Work out the finished part from the listing and answer in its coordinate system (mm). Face numbers are marked on the shaded views. A direction names the side the tool comes from. Coordinates: 2 decimals unless noted, no trailing zeros. Order: outer loops, then holes, each group sorted by start corner. A loop starts at its lowest first (then second) coordinate and runs counter-clockwise, first axis right, second up. Notation, with made-up numbers: M 22,22.25 L 36,22.25 A14 ccw 36,33.25 Z; hole C 68,-29.5 d5. An arc over 180 degrees is marked long. Use a Markdown table: item, result.
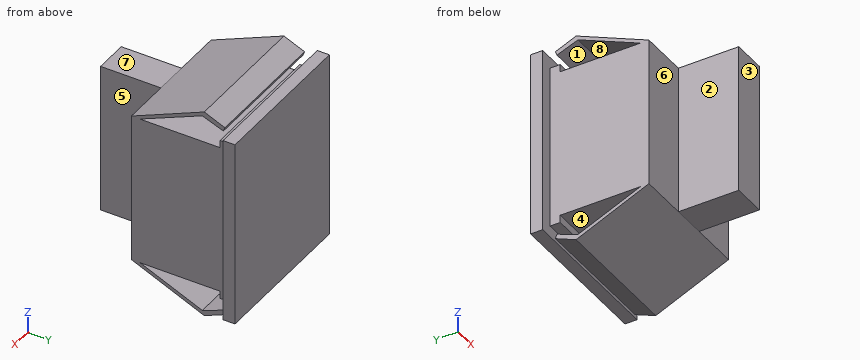
from build123d import *

# Parameters (mm, degrees)
EXTRUDE_1_DEPTH          = 25.6
SKETCH_2_OUTSIDE_W       = 38.032
SKETCH_2_OUTSIDE_H       = 40.832
CUT_EXTRUDE_1_DEPTH      = 6.235907328
CUT_EXTRUDE_1_DEPTH_BACK = 31.235907328


with BuildPart() as part:
    # Эскиз1 → Бобышка-Вытянуть1 (new body)
    with BuildSketch(Plane(origin=(0, 0, 0), x_dir=(0, 0, -1), z_dir=(1, 0, 0))):
        Polygon((12.5, 0), (-12.5, 0), (-12.5, 10), (-17.735907328, 22.085646779), (-16.27222348, 25.510475942), (-15.6, 25.25148825), (-16.94444696, 21.761867538), (-12.5, 11.400931817), (-12.5, 24.709221845), (-13.75, 24.709221845), (-13.75, 26.4), (-15.6, 26.4), (-15.6, 28.4), (15.6, 28.4), (15.6, 26.4), (13.75, 26.4), (13.75, 24.709221845), (12.5, 24.709221845), (12.5, 11.400931817), (16.94444696, 21.761867538), (15.6, 25.25148825), (16.27222348, 25.510475942), (17.735907328, 22.085646779), (12.5, 10), align=None)
    extrude(amount=EXTRUDE_1_DEPTH)

    # Эскиз2 outside → Вырез-Вытянуть1 (cut, two sides)
    with BuildSketch(Plane.XY.offset(12.5)) as cut_extrude_1_sk:
        with Locations((12.8, 14.2)):
            Rectangle(SKETCH_2_OUTSIDE_W, SKETCH_2_OUTSIDE_H)
        Polygon((2, 10), (2, 26.4), (0, 26.4), (0, 28.4), (25.6, 28.4), (25.6, 26.4), (23.6, 26.4), (23.6, 10), (15.6, 10), (15.6, 0), (10, 0), (10, 10), align=None, mode=Mode.SUBTRACT)
    extrude(amount=CUT_EXTRUDE_1_DEPTH, mode=Mode.SUBTRACT)
    extrude(cut_extrude_1_sk.sketch, amount=-CUT_EXTRUDE_1_DEPTH_BACK, mode=Mode.SUBTRACT)


solid = part.part
1. For the marked faces 5, 6, 7 and 8, determine the directions among +Z, -Z, +X, -X, +Y, -Y from which every point of the face is accessible in a straight line to the end or side of a thin tool.
Answers below:
| item | result |
|---|---|
| face 5 | +Z, -Z, +X, -Y |
| face 6 | +Z, -Z, -X, -Y |
| face 7 | +Z, +X, -X, -Y |
| face 8 | +X, -X |
2. Section D-D on z = 0 is taken. Determine the outline of the cut face in (x, y).
Answers below:
| item | result |
|---|---|
| outline | M 0,26.4 L 2,26.4 L 2,10 L 10,10 L 10,0 L 15.6,0 L 15.6,10 L 23.6,10 L 23.6,26.4 L 25.6,26.4 L 25.6,28.4 L 0,28.4 Z |
3. Flat-ended cylindrical pins translate along their axes: P1, Ø3, axis at y = 22, z = 9.5, coming from the -X side; P2, Ø0.6, axis at x = 16.5, y = 27.5, coming from the +Z side; P3, Ø6, axis at y = 3, z = 5.5, coming from the -X side; P4, Ø6.5, axis at x = 18.5, z = 3, coming from the -Y side. Find the tip coordinate at first contact, or state that the pin passes through.
Answers below:
| item | result |
|---|---|
| P1 | x = 2 |
| P2 | z = 15.6 |
| P3 | x = 10 |
| P4 | y = 0 |
4. For a pull along Y with two mould halves and no side action, classify the marked faces 1, 2, 3 and 4 as +Y half, -Y half, draft (parallel to the pull), parting line (faces both ways), or undercut.
Answers below:
| item | result |
|---|---|
| face 1 | undercut |
| face 2 | draft |
| face 3 | -Y half |
| face 4 | undercut |
5. Section C-C on y = 18.25 is taken. Determine the outline of the cut face in (x, z).
Answers below:
| item | result |
|---|---|
| outline | M 2,-16.07 L 23.6,-16.07 L 23.6,-15.44 L 2,-15.44 Z; M 2,-12.5 L 23.6,-12.5 L 23.6,12.5 L 2,12.5 Z; M 2,15.44 L 23.6,15.44 L 23.6,16.07 L 2,16.07 Z |
6. Section B-B on x = 14.25 is taken. Determine the outline of the cut face in (y, z).
Answers below:
| item | result |
|---|---|
| outline | M 0,-12.5 L 10,-12.5 L 22.09,-17.74 L 25.51,-16.27 L 25.25,-15.6 L 21.76,-16.94 L 11.4,-12.5 L 24.71,-12.5 L 24.71,-13.75 L 26.4,-13.75 L 26.4,-15.6 L 28.4,-15.6 L 28.4,15.6 L 26.4,15.6 L 26.4,13.75 L 24.71,13.75 L 24.71,12.5 L 11.4,12.5 L 21.76,16.94 L 25.25,15.6 L 25.51,16.27 L 22.09,17.74 L 10,12.5 L 0,12.5 Z |
7. Section A-A on z = -13 is taken. Determine the outline of the cut face in (x, y).
Answers below:
| item | result |
|---|---|
| outline | M 0,26.4 L 2,26.4 L 2,24.71 L 23.6,24.71 L 23.6,26.4 L 25.6,26.4 L 25.6,28.4 L 0,28.4 Z; M 2,11.15 L 23.6,11.15 L 23.6,12.57 L 2,12.57 Z |
8. Find the intervals of material crossed by probe 1 along Z at (x, y) = (13.25, 22.25); probe 2 along Z at (x, y) = (13.25, 15); probe 3 along X at (y, z) = (7, 11.5), in increasing order.
Answers below:
| item | result |
|---|---|
| probe 1 | -17.67 to -16.76, -12.5 to 12.5, 16.76 to 17.67 |
| probe 2 | -14.67 to -14.04, -12.5 to 12.5, 14.04 to 14.67 |
| probe 3 | 10 to 15.6 |
